Could you check a few things on this model? Use its own coordinates, in mm. Face numbers are marked on the shaded views. Round coordinates to 2 decimals unless told otherwise and drop trailing zeros. Order: outer loops, then holes, each group sorted by start corner. A loop starts at its lowest first (then second) coordinate and runs counter-clockwise, first axis right, second up.
Autodesk Fusion 360 part; units mm, degrees
sketch "Sketch1" plane through (0, 0, 0) normal (0, 0, 1) x (1, 0, 0)
  circle A0 centre (0, 0) radius 10
  dimension "d1" = 20
extrude "Extrude1" add sketch "Sketch1" along normal blind 25
sketch "Sketch2" plane through (0, 0, 25) normal (0, 0, 1) x (-1, 0, 0)
  circle A0 centre (0, 0) radius 10
  circle A1 centre (0, 0) radius 1.5
  dimension "d4" = 3
extrude "Extrude2" cut sketch "Sketch2" against normal blind 20 contours A1
chamfer "Chamfer1" distance 1 angle 45 2 faces at (7.1294, -0.4968, 25) (2.3712, -3.5556, 0)
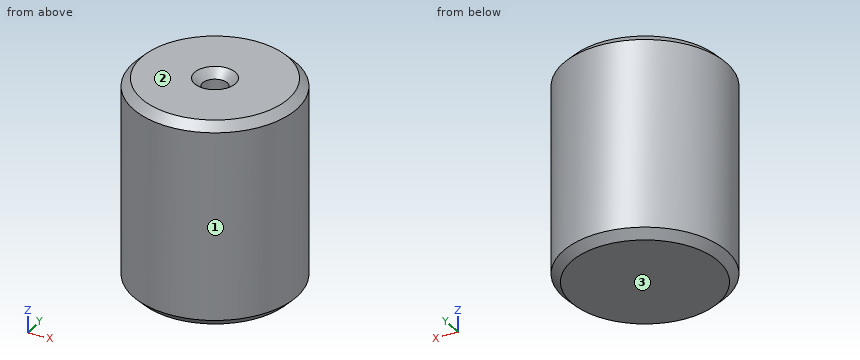
Q1. We'd pull the mould along Z, two halves only. Please class the marked faces 1, 2 and 3: released by +Z, released by -Z, zero draft, split by the parting line, or undercut.
Q2. Imagine slicing it at A-A, the plane y = 0. Please give me the cut outline in (x, z), then the cut area to 3 significant figures.
Q3. I need wall thicknesses on L1, parallel to Y at x = 0, z = 16.5; L2, parallel to X at y = 0.5, z = 9; L3, parallel to X at y = 2, z = 8. Which ranges of each line are inside material? Lowest first, please.
Q4. Imagine slicing it at C-C, the plane z = 8.25. Please give me the cut outline in (x, y).
Q5. For P1, Ø4, axis at x = 4, z = 22, coming from the -Y side; P2, Ø3.5, axis at x = 0, y = 0, coming from the +Z side; P3, Ø6, axis at x = 3.5, z = 6, coming from the +Y side; P4, Ø10, axis at x = 2.5, z = 18.5, coming from the -Y side, each with a flat end and sliding along its axis, tell me the tip position at first contact or that it passes through.
Filled in:
1. face 1: zero draft
1. face 2: released by +Z
1. face 3: released by -Z
2. outline: (-10, 1) - (-9, 0) - (9, 0) - (10, 1) - (10, 24) - (9, 25) - (2.5, 25) - (1.5, 24) - (1.5, 5) - (-1.5, 5) - (-1.5, 24) - (-2.5, 25) - (-9, 25) - (-10, 24) - close
2. area: 437 mm2
3. L1: y = -10 to -1.5, 1.5 to 10
3. L2: x = -9.99 to -1.41, 1.41 to 9.99
3. L3: x = -9.8 to 9.8
4. outline: circle Ø20 at (0, 0); hole circle Ø3 at (0, 0)
5. P1: stops at y = -9.8
5. P2: stops at z = 24.25
5. P3: stops at y = 9.99
5. P4: stops at y = -10
